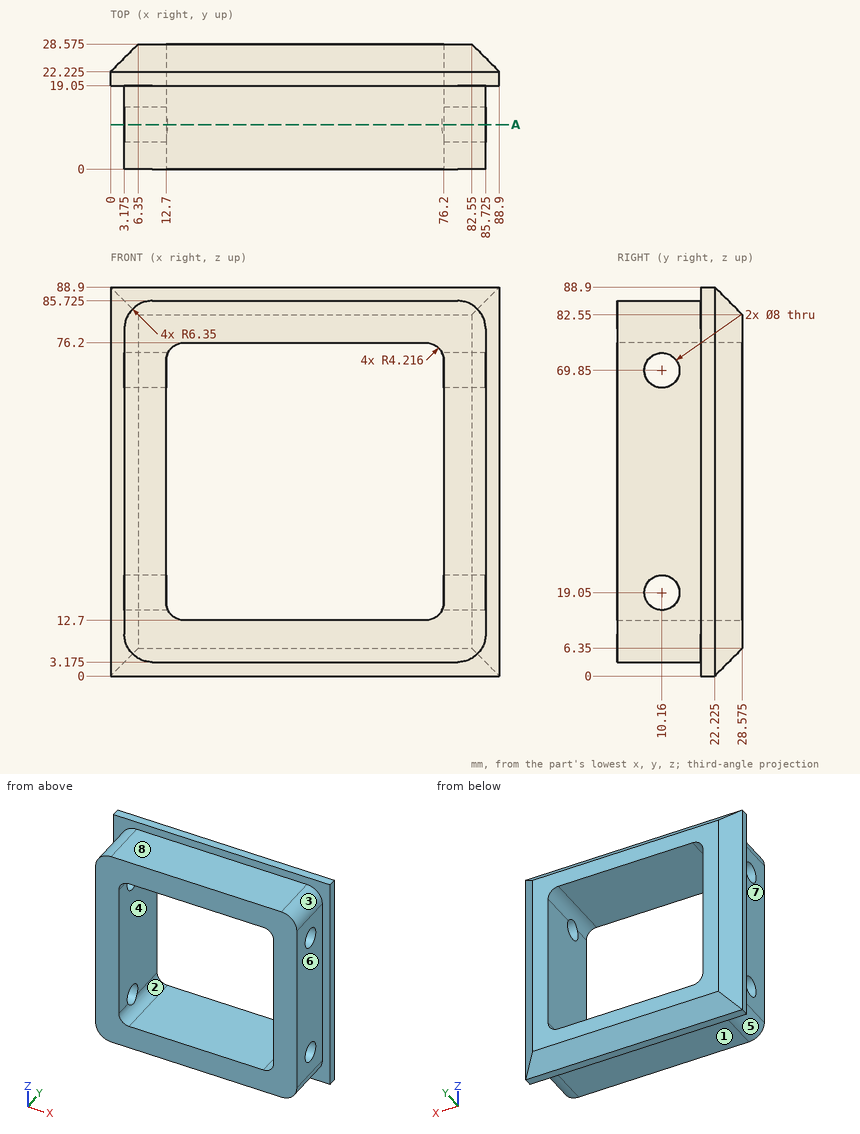
Study the drawing (mm; zero at the part's minimum x, y, z) and answer. A direction names the side the tool comes from. Give positions to 0.01 mm unless a question says otherwise; leave off trailing zeros.
(1) The part is cut by section A-A on y = 10.16. Count the separate pieces of the cut face and the enclosed holes in it, plus the area to 3 significant figures.
Final values:
separate pieces: 4
enclosed holes: 0
area: 2,460 mm2
(2) Straight lines are drawn through the part: line 1 (X direction, y = 17.75, z = 55.5) (1 decimal); line 2 (Z direction, x = 7.5, y = 10.16); line 3 (Y direction, x = 82, z = 19.05) (1 decimal). For each, find the intervals that lie inside material, in ascending order.
Final values:
line 1: x = 3.2 to 12.7, 76.2 to 85.7
line 2: z = 3.51 to 15.05, 23.05 to 65.85, 73.85 to 85.39
line 3: y = 0 to 6.2, 14.2 to 28.6
(3) Flat-ended cylindrical pins translate along their axes: pin 1 Ø10 at (y, z) = (9.5, 32.5) entering from -X (3 decimals); pin 2 Ø8.5 at (y, z) = (13, 46) entering from +X (3 decimals); pin 3 Ø5.5 at (x, y) = (42, 13) entering from +Z (3 decimals). Find the tip coordinate at first contact, or state that the pin passes through.
Final values:
pin 1: stops at x = 3.175
pin 2: stops at x = 85.725
pin 3: stops at z = 85.725
(4) The mould has two halves that part along X. Classify the marked faces 1, 2 and 3: pulls with the +X half, pulls with the -X half, needs draft (parallel to the pull), parting line crosses it, or undercut.
Final values:
face 1: needs draft
face 2: undercut
face 3: pulls with the +X half
(5) Which of the six approach directions +Z, -Z, +X, -X, +Y, -Y give full straight-line access (tool end or side, diameter ignored) to the marked faces 4, 5, 6, 7 and 8?
Final values:
face 4: +Y, -Y
face 5: -Z, -X, -Y
face 6: +Z, -Z, +X, -Y
face 7: +Z, -Z, -X, -Y
face 8: +Z, +X, -X, -Y
